Design review of the part shown in the three views and the two pictorial views. Dimensions are in mm from the part's minimum x, y and z. Coordinates: 2 decimals unless noted, no trailing zeros. Write each loop counter-clockwise with the first axis right and the second up, starting at its lowest first coordinate (ties: lowest second). Pieces come first, ordered by that corner, then holes. Notation, with made-up numbers: M -10.5,2.25 L 41.5,2.25 A19 ccw 41.5,23.25 Z; hole C 50,-15.75 d11. An arc over 180 degrees is marked long. Answer as a JSON object with one key per item and string values.
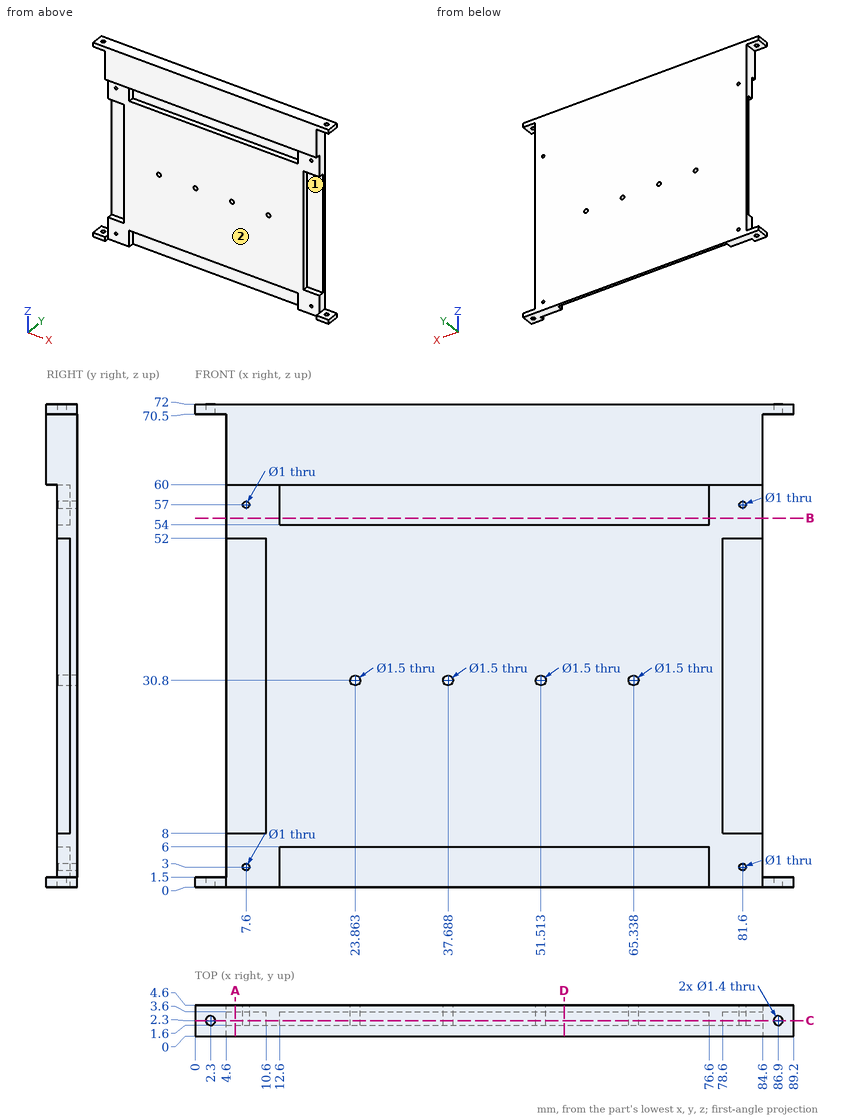
(1) For pin 1 Ø1 at (y, z) = (2.5, 58) entering from -X; pin 2 Ø2 at (x, z) = (51.51, 30.8) entering from -Y; pin 3 Ø1.4 at (x, y) = (86, 1.5) entering from -Z; pin 4 Ø0.6 at (y, z) = (2.5, 2.5) entering from +X, all flat-tipped, find the tip position at first contact; note any pin that passes through.
Results list:
{"pin 1": "x = 4.6", "pin 2": "y = 1.6", "pin 3": "z = 0", "pin 4": "x = 84.6"}
(2) Add section B-B on z = 55. Give the boundary of the cut face in (x, y).
Results list:
{"outline": "M 4.6,1.6 L 12.6,1.6 L 12.6,3.6 L 76.6,3.6 L 76.6,1.6 L 84.6,1.6 L 84.6,4.6 L 4.6,4.6 Z"}
(3) Wall thickness on line 1 along Z through (x, y) = (81.6, 2.7); line 2 along X through (y, z) = (3, 3); line 3 along Y through (x, z) = (86.9, 71.1): over which ranges is each line inside the solid? List them lowest first. Write a range as from..to.
Results list:
{"line 1": "0..2.5, 3.5..8, 52..56.5, 57.5..72", "line 2": "4.6..7.1, 8.1..12.6, 76.6..81.1, 82.1..84.6", "line 3": "0..1.6, 3..4.6"}
(4) Add section A-A on x = 6. Give the boundary of the cut face in (y, z).
Results list:
{"outline": "M 0,60 L 1.6,60 L 1.6,52 L 3.6,52 L 3.6,8 L 1.6,8 L 1.6,0 L 4.6,0 L 4.6,72 L 0,72 Z"}
(5) Draft analysis for pull direction Z (two halves, no side actions). For the marked faces 1 and 2, state which applies: released by +Z, released by -Z, zero draft, split by the parting line, or undercut.
Results list:
{"face 1": "undercut", "face 2": "zero draft"}
(6) Add section D-D on x = 55. Give the boundary of the cut face in (y, z), and give its area (3 significant figures).
Results list:
{"outline": "M 0,60 L 3.6,60 L 3.6,54 L 1.6,54 L 1.6,6 L 3.6,6 L 3.6,0 L 4.6,0 L 4.6,72 L 0,72 Z", "area": "211 mm²"}
(7) Add section C-C on y = 2.3. Count the separate pieces of the cut face and the enclosed holes in it, and give its area (3 significant figures).
Results list:
{"separate pieces": "5", "enclosed holes": "9", "area": "4,470 mm²"}
